from build123d import *

# Parameters (mm, degrees)
F0_R     = 22.25
F0_R_2   = 19.75
F1_DEPTH = 7


# Not quite as in the source:
# - a feature of the source that left no trace in its solid (it failed there, or was rolled back) is left out
# - the program builds the solid bodies; features that only make, move or delete a surface that nothing else refers to are left out


with BuildPart() as f1:
    # F0 (on Front) → F1 (new body)
    with BuildSketch(Plane.XZ):
        Circle(F0_R)
        Circle(F0_R_2, mode=Mode.SUBTRACT)
    extrude(amount=F1_DEPTH)

    # F7 (on offset) → F8 (revolve, cut)
    with BuildSketch(Plane.YZ.offset(23)):
        with BuildLine():
            Line((-5.5, 0), (-1.5, 0))
            ThreePointArc((-1.5, 0), (-3.5, 2), (-5.5, 0))
        make_face()
    revolve(axis=Axis((23, -3.487871727, 0), (0, -1, 0)), mode=Mode.SUBTRACT)

    # F9: F1 across plane


with BuildPart() as f1_1:
    add(f1.part)
    add(f1.part.mirror(Plane.YZ), mode=Mode.INTERSECT)


solid = f1_1.part
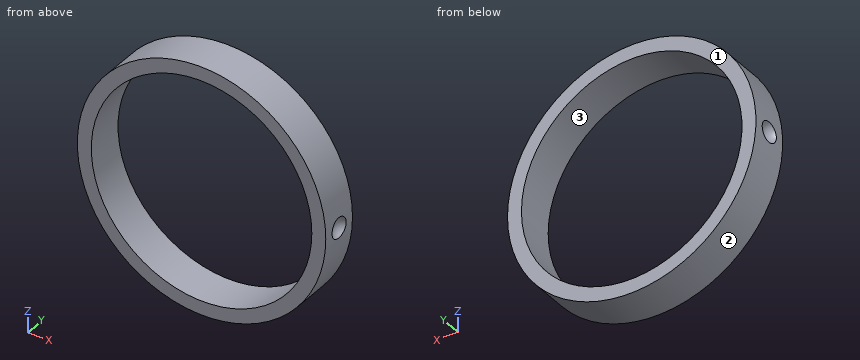
Read the model definition and answer for the solid it produces. Units are mm, in the model's axes. Face numbers are marked on the shaded views. Give positions to 0.01 mm unless a question says otherwise; leave off trailing zeros. Write each loop counter-clockwise with the first axis right and the second up, starting at its lowest first coordinate (ties: lowest second). Pieces come first, ordered by that corner, then holes. Notation, with made-up numbers: (74.5, 86) -> (101.5, 86) arc R22 cw to (101.5, 94) -> close; hole circle Ø10 at (-34.75, -11.5). An arc over 180 degrees is marked (long way). Answer as a JSON object with one key per item and string values. Group by question number.
1) Find section B-B (x = 0). Write down the section's boundary in (y, z), and give its area (3 significant figures).
2) Find section C-C (y = -4). Write down the section's boundary in (x, z).
3) Find section A-A (z = 0). Write down the section's boundary in (x, y), and give its area (3 significant figures).
4) Each of these flat-tipped pins is pushed along its axis until it touches: P1, Ø3, axis at y = -1, z = -7, coming from the +X side; P2, Ø2, axis at x = -13, y = -3, coming from the -Z side; P3, Ø1, axis at y = -4.5, z = -3.5, coming from the +X side; P4, Ø23.5, axis at x = 0, z = 0, coming from the +Y side. Where does it stop, or does it pass through?
5) The mould has two halves that part along X. Classify the marked faces 1, 2 and 3: +X half, -X half, draft (parallel to the pull), parting line (faces both ways), or undercut.
6) Consider L1, parallel to Z at x = 0, y = -2.25; L2, parallel to X at y = -2.25, z = 5. Determine where each line is inside the solid, lowest interval first. Write a range as from..to.
7) Find section D-D (x = -6). Write down the section's boundary in (y, z), and give its area (3 significant figures).
Values follow:
{
 "1": {"outline": "(-7, -22.25) -> (0, -22.25) -> (0, -19.75) -> (-7, -19.75) -> close; (-7, 19.75) -> (0, 19.75) -> (0, 22.25) -> (-7, 22.25) -> close", "area": "35.0 mm2"},
 "2": {"outline": "(-22.18, -1.75) arc R22.25 ccw to (22.18, -1.75) arc R1.94 cw to (22.18, 1.75) arc R22.25 ccw to (-22.18, 1.75) arc R1.94 cw to start; hole circle Ø39.5 at (0, 0)"},
 "3": {"outline": "(-22.25, -7) -> (-19.75, -7) -> (-19.75, 0) -> (-22.25, 0) -> (-22.25, -1.65) arc R2 cw to (-22.25, -5.35) -> close; (19.75, -7) -> (22.25, -7) -> (22.25, -5.35) arc R2 cw to (22.25, -1.65) -> (22.25, 0) -> (19.75, 0) -> close", "area": "28.3 mm2"},
 "4": {"P1": "stops at x = 21.56", "P2": "stops at z = -18.74", "P3": "stops at x = 22.05", "P4": "passes through"},
 "5": {"face 1": "draft", "face 2": "parting line", "face 3": "undercut"},
 "6": {"L1": "z = -22.25..-19.75, 19.75..22.25", "L2": "x = -21.68..-19.11, 19.11..21.68"},
 "7": {"outline": "(-7, -21.43) -> (0, -21.43) -> (0, -18.82) -> (-7, -18.82) -> close; (-7, 18.82) -> (0, 18.82) -> (0, 21.43) -> (-7, 21.43) -> close", "area": "36.5 mm2"}
}
